Here's the drawing with two shaded views (mm, measured from the low corner). I have some questions. A direction names the side the tool comes from. Give positions to 0.01 mm unless a question says otherwise; leave off trailing zeros. Loops run counter-clockwise (first coordinate to the right, second up) from the corner with the lowest first, then second, coordinate; pieces in that order, holes last. Notation, with made-up numbers: (-1.75, 24.5) - (46.25, 24.5) arc R17 cw to (46.25, 29.5) - close; hole circle Ø8 at (14.25, -17). An arc over 180 degrees is marked (long way). Write each question's results on one line, items separated by ' | '. Start each with the question number.
1) I want a section at C-C, the plane x = 37. Write out the boundary of the cut face in (y, z).
2) I want a section at A-A, the plane x = 60.5. Write out the boundary of the cut face in (y, z) (1 decimal).
3) If we mould it in two halves opening along Y, with no side actions, what happens to the marked faces 1, 2, 3 and 4? For each: +Y half, -Y half, draft (parallel to the pull), parting line (faces both ways), or undercut.
4) I want a section at D-D, the plane z = 24. Write out the boundary of the cut face in (x, y).
5) I want a section at B-B, the plane y = 34.5. Write out the boundary of the cut face in (x, z).
6) If I drill on probe 1 along X at (y, z) = (25, 40) (1 decimal); probe 2 along X at (y, z) = (26, 26); probe 3 along X at (y, z) = (43.5, 10.5), over which ranges is the centre line in solid material (lowest first)? Write a range as [from, to].
7) On a 3-axis mill with a long thin cutter (end or side, diameter ignored), from which of +Z, -Z, +X, -X, +Y, -Y can I reach the whole of each face in a straight line? I mean the marked faces 5, 6, 7, 8 and 9. Say none if no direction works.
8) I'm going to push flat-ended pins straight in: pin 1 (5 mm diameter, centred on y = 9.5, z = 8, fed in from +X); pin 2 (11.5 mm diameter, centred on x = 19.05, y = 29.591, fed in from -Z); pin 3 (3 mm diameter, centred on x = 43.5, z = 45, fed in from +Y); pin 4 (20.5 mm diameter, centred on x = 57.15, y = 29.591, fed in from +Z). Where does each tip first touch, or does it pass through?
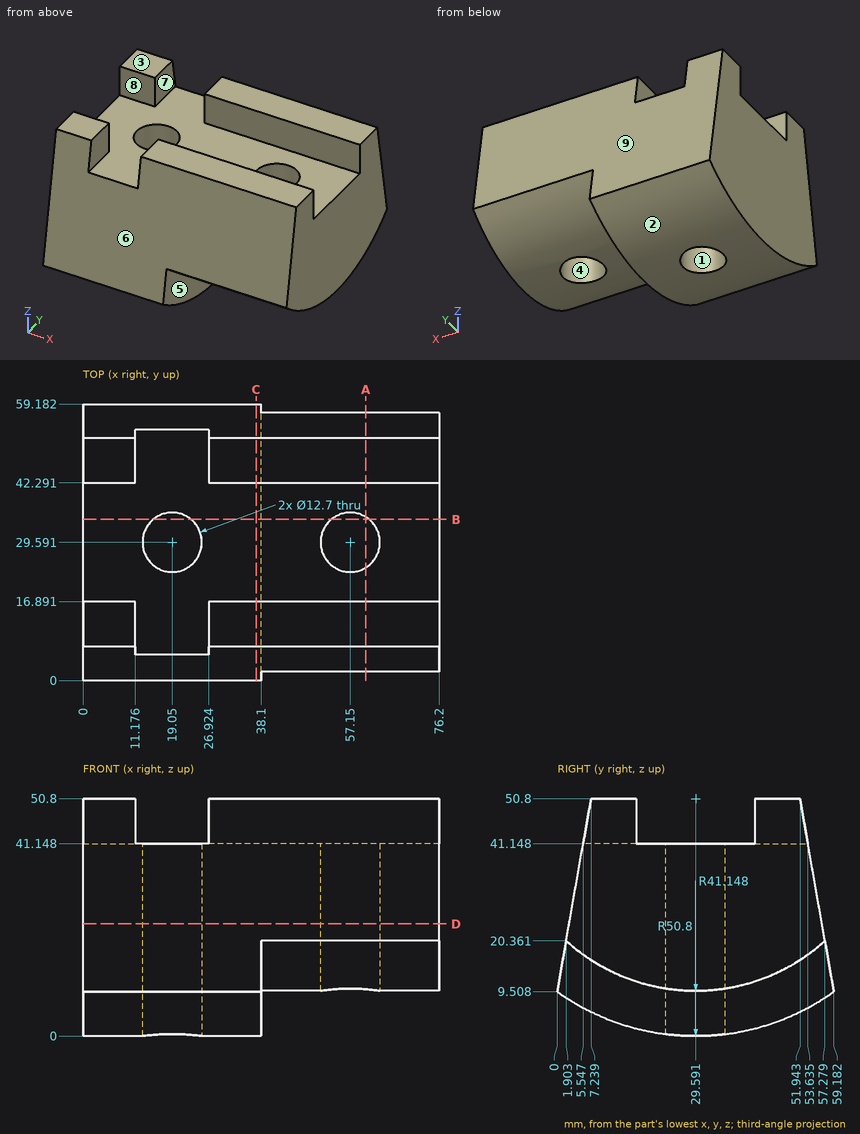
Answers:
1) outline: (0, 9.51) arc R50.8 ccw to (59.18, 9.51) - (51.94, 50.8) - (42.29, 50.8) - (42.29, 41.15) - (16.89, 41.15) - (16.89, 50.8) - (7.24, 50.8) - close
2) outline: (1.9, 20.4) arc R41.1 ccw to (24.2, 10) - (24.2, 41.1) - (16.9, 41.1) - (16.9, 50.8) - (7.2, 50.8) - close; (35, 10) arc R41.1 ccw to (57.3, 20.4) - (51.9, 50.8) - (42.3, 50.8) - (42.3, 41.1) - (35, 41.1) - close
3) face 1: undercut | face 2: parting line | face 3: draft | face 4: undercut
4) outline: (0, 2.54) - (76.2, 2.54) - (76.2, 56.64) - (0, 56.64) - close; hole circle Ø12.7 at (19.05, 29.59); hole circle Ø12.7 at (57.15, 29.59)
5) outline: (0, 0.24) - (15.02, 0.24) - (15.02, 41.15) - (0, 41.15) - close; (23.08, 0.24) - (38.1, 0.24) - (38.1, 9.95) - (53.12, 9.95) - (53.12, 41.15) - (23.08, 41.15) - close; (61.18, 9.95) - (76.2, 9.95) - (76.2, 41.15) - (61.18, 41.15) - close
6) probe 1: x = [0, 14.7], [23.4, 52.8], [61.5, 76.2] | probe 2: x = [0, 13.81], [24.29, 51.91], [62.39, 76.2] | probe 3: x = [0, 38.1]
7) face 5: -Z, +X | face 6: +Z, +X, -X, -Y | face 7: +Z, +Y, -Y | face 8: +Z, +X, -X | face 9: +Z, +X, -X, +Y
8) pin 1: stops at x = 38.1 | pin 2: passes through | pin 3: stops at y = 53.22 | pin 4: stops at z = 41.15
